from build123d import *

# Parameters (mm, degrees)
SKETCH1_R           = 1.5
BOSS_EXTRUDE1_DEPTH = 3


with BuildPart() as part:
    # Sketch1 → Boss-Extrude1 (new body)
    with BuildSketch(Plane(origin=(0, 0, 0), x_dir=(1, 0, 0), z_dir=(0, 1, 0))):
        with BuildLine():
            ThreePointArc((-21.904580175, -11.149573826), (-16.613262981, 7.314570744), (2.310408028, 4.025597064))
            Line((2.310408028, 4.025597064), (6.530490254, -4.452553635))
            Line((6.530490254, -4.452553635), (15.07165127, 9.857606543))
            ThreePointArc((15.07165127, 9.857606543), (-16.700482533, 9.891564727), (-32.623744859, -17.602422915))
            Line((-32.623744859, -17.602422915), (-19.537696929, -19.565138538))
            Line((-19.537696929, -19.565138538), (-21.904580175, -11.149573826))
        make_face()
        with Locations(Location((-23.321800839, -14.928602489, 0), (0, 0, 270))):
            Circle(SKETCH1_R, mode=Mode.SUBTRACT)
        with Locations(Location((6.377238608, 3.590767262, 0), (0, 0, 270))):
            Circle(SKETCH1_R, mode=Mode.SUBTRACT)
    extrude(amount=BOSS_EXTRUDE1_DEPTH)


solid = part.part
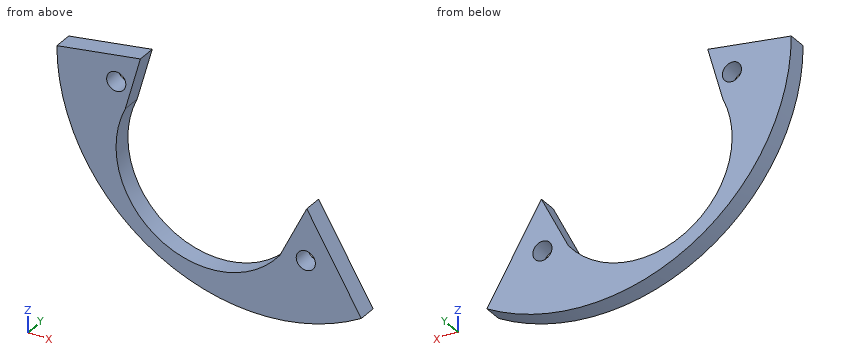
Can you work these out from the model? Positions are in its coordinate system, mm. Round coordinates to 2 decimals unless told otherwise and drop trailing zeros. Write each loop counter-clockwise with the first axis right and the second up, starting at its lowest first coordinate (ties: lowest second). Pieces come first, ordered by that corner, then holes. Notation, with made-up numbers: M -26.75,-19.5 L -22.75,-19.5 A18 ccw -22.75,-3.5 Z; hole C 42.25,27.25 d10. An arc over 180 degrees is marked long. Use CSV: the item, a comma, the result in double quotes.
(1) I'm going to push flat-ended pins straight in: pin 1 (1 mm diameter, centred on y = 2.5, z = -10.5, fed in from -X); pin 2 (1.5 mm diameter, centred on x = -23, y = 0.5, fed in from -Z); pin 3 (1 mm diameter, centred on x = 4.5, y = 1.5, fed in from -Z). Where does each tip first touch, or does it pass through?
Check values:
pin 1,"x = -16.51"
pin 2,"z = -5.84"
pin 3,"z = -13.76"
(2) Imagine slicing it at C-C (y = 1.05). Write out the boundary of the cut face in (x, z), plus the area to 3 significant figures.
Check values:
outline,"M -32.62,17.6 A31.78 ccw 15.07,-9.86 L 6.53,4.45 L 2.31,-4.03 A14.37 cw -21.9,11.15 L -19.54,19.57 Z; hole C -23.32,14.93 d3; hole C 6.38,-3.59 d3"
area,"412 mm^2"
(3) Imagine slicing it at B-B (x = -24). Write out the boundary of the cut face in (y, z), plus the area to 3 significant figures.
Check values:
outline,"M 0,-4.12 L 3,-4.12 L 3,13.59 L 0,13.59 Z; M 0,16.27 L 3,16.27 L 3,18.9 L 0,18.9 Z"
area,"61.0 mm^2"
(4) I need wall thicknesses on line 1 along X through (y, z) = (2.55, -4); line 2 along X through (y, z) = (1.05, -3); line 3 along X through (y, z) = (2.65, 1.5). Which ranges of each line are inside material? Lowest first, please.
Check values:
line 1,"-24.11 to -20.29, 2.32 to 4.93, 7.82 to 11.58"
line 2,"-25 to -21.01, 2.82 to 5, 7.76 to 10.98"
line 3,"-28.21 to -22.95, 5.06 to 8.29"
(5) Imagine slicing it at D-D (z = 12.5). Write out the boundary of the cut face in (x, y).
Check values:
outline,"M -32.2,0 L -21.52,0 L -21.52,3 L -32.2,3 Z"
(6) Imagine slicing it at A-A (z = -7). Write out the boundary of the cut face in (x, y).
Check values:
outline,"M -20.9,0 L -17.09,0 L -17.09,3 L -20.9,3 Z; M -0.87,0 L 13.37,0 L 13.37,3 L -0.87,3 Z"
